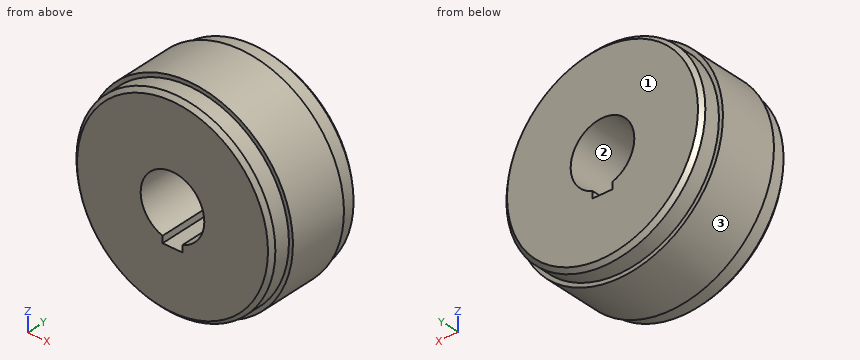
from build123d import *

# Parameters (mm, degrees)
SKETCH_1_R      = 25
EXTRUDE_1_DEPTH = 12.5
SKETCH_2_R      = 26
SKETCH_2_R_2    = 24
EXTRUDE_2_DEPTH = 7.5
CHAMFER_1_SIZE  = 1


with BuildPart() as part:
    # 草图1 → 凸台-拉伸1 (new, symmetric)
    with BuildSketch(Plane(origin=(0, 0, 0), x_dir=(1, 0, 0), z_dir=(0, 1, 0))):
        with Locations(Location((0, 0, 0), (0, 0, 270))):
            Circle(SKETCH_1_R)
        with BuildLine():
            Line((-2.5, 7.599342077), (-2.5, 9.3))
            Line((-2.5, 9.3), (2.5, 9.3))
            Line((2.5, 9.3), (2.5, 7.599342077))
            ThreePointArc((2.5, 7.599342077), (0, -8), (-2.5, 7.599342077))
        make_face(mode=Mode.SUBTRACT)
    extrude(amount=EXTRUDE_1_DEPTH, both=True)

    # 草图2 → 凸台-拉伸2 (add, symmetric)
    with BuildSketch(Plane(origin=(0, 0, 0), x_dir=(1, 0, 0), z_dir=(0, 1, 0))):
        with Locations(Location((0, 0, 0), (0, 0, 270))):
            Circle(SKETCH_2_R)
        Circle(SKETCH_2_R_2, mode=Mode.SUBTRACT)
    extrude(amount=EXTRUDE_2_DEPTH, both=True)

    # 倒角1
    chamfer_1_edges = [part.edges().sort_by_distance(p)[0] for p in [
        (0, -12.5, -25),
        (0, 12.5, -25),
    ]]
    chamfer(chamfer_1_edges, length=CHAMFER_1_SIZE)


solid = part.part
Build history of the part. All positions in model axes, mm. Face numbers are marked on the shaded views. Coordinates: 2 decimals unless noted, no trailing zeros. Write each loop counter-clockwise with the first axis right and the second up, starting at its lowest first coordinate (ties: lowest second). Pieces come first, ordered by that corner, then holes.
(1) Pin check, flat tips, straight feed: pin 1 Ø5 at (y, z) = (0, -3.5) entering from -X; pin 2 Ø2 at (x, y) = (15, 7) entering from -Z; pin 3 Ø5.5 at (x, y) = (-0.5, 4.5) entering from +Z; pin 4 Ø10 at (y, z) = (-4, 20.5) entering from -X. Stop position of each tip, or through.
(2) Cut at C-C on x = 0. List the corners of the cut face in (y, z), and give its area (4 significant figures).
(3) Cut at A-A on z = 0. List the corners of the cut face in (x, y), and give its area (3 significant figures).
(4) Drill centre lines: line 1 (X direction, y = -4.5, z = 0); line 2 (X direction, y = -7.75, z = 0.5) (3 decimals); line 3 (Z direction, x = -6, y = -4.25). Where is each one in solid material? Low to high.
(5) Cut at B-B on y = -2. List the corners of the cut face in (x, z).
(6) Mould opens along Z. For the marked faces 1, 2 and 3 say: pulls with the +Z half, pulls with the -Z half, needs draft (parallel to the pull), parting line crosses it, or undercut.
(7) Cut at D-D on y = -9.5. List the corners of the cut face in (x, z).
Working result:
1. pin 1: stops at x = -25.98
1. pin 2: stops at z = -21.91
1. pin 3: stops at z = 26
1. pin 4: stops at x = -20.87
2. outline: (-12.5, -24) - (-11.5, -25) - (-7.5, -25) - (-7.5, -26) - (7.5, -26) - (7.5, -25) - (11.5, -25) - (12.5, -24) - (12.5, -9.3) - (-12.5, -9.3) - close; (-12.5, 8) - (12.5, 8) - (12.5, 24) - (11.5, 25) - (7.5, 25) - (7.5, 26) - (-7.5, 26) - (-7.5, 25) - (-11.5, 25) - (-12.5, 24) - close
2. area: 845.5 mm2
3. outline: (-26, -7.5) - (-25, -7.5) - (-25, -11.5) - (-24, -12.5) - (-8, -12.5) - (-8, 12.5) - (-24, 12.5) - (-25, 11.5) - (-25, 7.5) - (-26, 7.5) - close; (8, -12.5) - (24, -12.5) - (25, -11.5) - (25, -7.5) - (26, -7.5) - (26, 7.5) - (25, 7.5) - (25, 11.5) - (24, 12.5) - (8, 12.5) - close
3. area: 878 mm2
4. line 1: x = -26 to -8, 8 to 26
4. line 2: x = -24.995 to -7.984, 7.984 to 24.995
4. line 3: z = -25.3 to -5.29, 5.29 to 25.3
5. outline: circle Ø52 at (0, 0); hole (-2.5, -9.3) - (2.5, -9.3) - (2.5, -7.6) arc R8 ccw (long way) to (-2.5, -7.6) - close
6. face 1: needs draft
6. face 2: undercut
6. face 3: parting line crosses it
7. outline: circle Ø50 at (0, 0); hole (-2.5, -9.3) - (2.5, -9.3) - (2.5, -7.6) arc R8 ccw (long way) to (-2.5, -7.6) - close
